Check sheet for the modelled part. Datum: model origin and axes. Units: mm. A direction names the side the tool comes from. Give positions to 0.01 mm unless a question says otherwise; leave off trailing zeros. Order: outer loops, then holes, each group sorted by start corner. A loop starts at its lowest first (then second) coordinate and runs counter-clockwise, first axis right, second up. Notation, with made-up numbers: (68.5, 40) -> (111.5, 40) arc R26 cw to (111.5, 64) -> close; hole circle Ø4 at (73.25, 88). An arc over 180 degrees is marked (long way). Answer in a Markdown table with one row per item. Add a question column.
(1) Thickness scan on L1, parallel to Y at x = 0, z = 1.5; L2, parallel to Z at x = -12.5, y = 11; L3, parallel to X at y = 5.25, z = 7. Record the ranges inside material, lowest first. Write a range as [from, to].
(2) Cross-section at B-B (y = 0). Record the cut outline in (x, z), then the cut area to 3 significant figures.
(3) Cross-section at C-C (z = 13). Record the cut outline in (x, y).
(4) Release check for a two-part mould opening along Z. For faces 1 (the face through (0, -12, 7)), 2 (the face through (-0.54, -2.44, 12.17)) record: released by +Z, released by -Z, zero draft, split by the parting line, or undercut.
(5) Set-up check for faces 3 (the face through (-1.84, -8.3, 19.07)), 4 (the face through (-2.437, 13.786, 7.07)), 5 (the face through (13.154, 4.794, 7.07)), 6 (the face through (-10.414, -5.964, 6.93)): record each of +Z, -Z, +X, -X, +Y, -Y from which the full face is reachable in a straight line by a thin tool's end or side.
(6) Cross-section at D-D (y = 6.5). Record the cut outline in (x, z).
(7) Cross-section at A-A (x = 0). Record the cut outline in (y, z).
(8) Go/stop test with flat-tipped pins: pin 1 (4 mm diameter, centred on x = 0, y = 0, fed in from -Z); pin 2 (10 mm diameter, centred on x = -13, y = 12, fed in from +Z); pin 3 (3.5 mm diameter, centred on x = 0, z = 19, fed in from -Y); pin 4 (4 mm diameter, centred on x = -13.5, z = 11, fed in from -Y). Record where each tip stops, or that it passes through.
```python
from build123d import *

# Parameters (mm, degrees)
SKETCH1_R                 = 17
BOSS_EXTRUDE1_DEPTH       = 14
CUT_EXTRUDE2_REACH        = 29.821
SKETCH3_R                 = 2.5
BOSS_EXTRUDE2_START       = 10
SKETCH5_R                 = 8.5
SKETCH5_R_2               = 2.5
BOSS_EXTRUDE2_DEPTH       = 10
SKETCH7_R                 = 17
SKETCH7_R_2               = 14
CUT_EXTRUDE5_DEPTH        = 5
SKETCH8_R                 = 2
CUT_EXTRUDE6_DEPTH        = 5
SKETCH9_R                 = 2
CUT_EXTRUDE7_DEPTH        = 10
M4_TAPPED_HOLE2_OUTLINE_W = 1.65
M4_TAPPED_HOLE2_OUTLINE_H = 10.992017373


with BuildPart() as part:
    # Sketch1 → Boss-Extrude1 (new body)
    with BuildSketch(Plane.XY):
        Circle(SKETCH1_R)
    extrude(amount=BOSS_EXTRUDE1_DEPTH)

    # Sketch3 → Cut-Extrude2 (cut, up to next)
    with BuildSketch(Plane.XY.offset(14), mode=Mode.PRIVATE) as cut_extrude2_sk1:
        Circle(SKETCH3_R)
    cut_extrude2_tool1 = extrude(cut_extrude2_sk1.sketch, amount=-CUT_EXTRUDE2_REACH, mode=Mode.PRIVATE) & part.part
    add(cut_extrude2_tool1.solids().sort_by_distance((0, 0, 14))[0], mode=Mode.SUBTRACT)

    # Sketch5 → Boss-Extrude2 (add)
    with BuildSketch(Plane.XY.offset(14).offset(BOSS_EXTRUDE2_START)):
        Circle(SKETCH5_R)
        Circle(SKETCH5_R_2, mode=Mode.SUBTRACT)
    extrude(amount=-BOSS_EXTRUDE2_DEPTH)

    # Sketch7 → Cut-Extrude5 (cut, symmetric)
    with BuildSketch(Plane(origin=(0, 0, 7), x_dir=(-1, 0, 0), z_dir=(0, 0, -1))):
        Circle(SKETCH7_R)
        Circle(SKETCH7_R_2, mode=Mode.SUBTRACT)
    extrude(amount=CUT_EXTRUDE5_DEPTH, both=True, mode=Mode.SUBTRACT)

    # Sketch8 → Cut-Extrude6 (cut, symmetric)
    with BuildSketch(Plane(origin=(0, 0, 7), x_dir=(-1, 0, 0), z_dir=(0, 0, -1))):
        with Locations((0, 14)):
            Circle(SKETCH8_R)
        with Locations((4.788282007, 13.155696691)):
            Circle(SKETCH8_R)
        with Locations((8.999026536, 10.724622204)):
            Circle(SKETCH8_R)
        with Locations((12.124355653, 7)):
            Circle(SKETCH8_R)
        with Locations((13.787308542, 2.431074487)):
            Circle(SKETCH8_R)
        with Locations((13.787308542, -2.431074487)):
            Circle(SKETCH8_R)
        with Locations((12.124355653, -7)):
            Circle(SKETCH8_R)
        with Locations((8.999026536, -10.724622204)):
            Circle(SKETCH8_R)
        with Locations((4.788282007, -13.155696691)):
            Circle(SKETCH8_R)
        with Locations((0, -14)):
            Circle(SKETCH8_R)
        with Locations((-4.788282007, -13.155696691)):
            Circle(SKETCH8_R)
        with Locations((-8.999026536, -10.724622204)):
            Circle(SKETCH8_R)
        with Locations((-12.124355653, -7)):
            Circle(SKETCH8_R)
        with Locations((-13.787308542, -2.431074487)):
            Circle(SKETCH8_R)
        with Locations((-13.787308542, 2.431074487)):
            Circle(SKETCH8_R)
        with Locations((-12.124355653, 7)):
            Circle(SKETCH8_R)
        with Locations((-8.999026536, 10.724622204)):
            Circle(SKETCH8_R)
        with Locations((-4.788282007, 13.155696691)):
            Circle(SKETCH8_R)
    extrude(amount=CUT_EXTRUDE6_DEPTH, both=True, mode=Mode.SUBTRACT)

    # Sketch9 → Cut-Extrude7 (cut)
    with BuildSketch(Plane(origin=(0, 0, 0), x_dir=(1, 0, 0), z_dir=(0, 1, 0))):
        with Locations(Location((0, -19, 0), (0, 0, 90))):
            Circle(SKETCH9_R)
    extrude(amount=CUT_EXTRUDE7_DEPTH, mode=Mode.SUBTRACT)

    # M4 Tapped Hole2: read off the stored shape, not the designer's step
    # M4 Tapped Hole2 outline → M4 Tapped Hole2 (revolve, cut)
    with BuildSketch(Plane.XY.offset(7)):
        with Locations((0.825, 7.373848872)):
            Rectangle(M4_TAPPED_HOLE2_OUTLINE_W, M4_TAPPED_HOLE2_OUTLINE_H)
    revolve(axis=Axis((0, 0, 7), (0, 1, 0)), mode=Mode.SUBTRACT)


solid = part.part
```
Answer below:
| question | item | result |
|---|---|---|
| 1 | L1 | y = [-17, -2.5], [2.5, 17] |
| 1 | L2 | z = [0, 2], [12, 14] |
| 1 | L3 | x = [-11.16, -1.65], [1.65, 11.16] |
| 2 | outline | (-17, 0) -> (-2.5, 0) -> (-2.5, 24) -> (-8.5, 24) -> (-8.5, 14) -> (-17, 14) -> (-17, 12) -> (-14, 12) -> (-14, 2) -> (-17, 2) -> close; (2.5, 0) -> (17, 0) -> (17, 2) -> (14, 2) -> (14, 12) -> (17, 12) -> (17, 14) -> (8.5, 14) -> (8.5, 24) -> (2.5, 24) -> close |
| 2 | area | 466 mm² |
| 3 | outline | circle Ø34 at (0, 0); hole circle Ø5 at (0, 0) |
| 4 | face 1 | undercut |
| 4 | face 2 | zero draft |
| 5 | face 3 | +Z |
| 5 | face 4 | -X, +Y |
| 5 | face 5 | +X, +Y |
| 5 | face 6 | none |
| 6 | outline | (-15.71, 0) -> (15.71, 0) -> (15.71, 2) -> (10.19, 2) -> (10.19, 12) -> (15.71, 12) -> (15.71, 14) -> (5.48, 14) -> (5.48, 24) -> (-5.48, 24) -> (-5.48, 14) -> (-15.71, 14) -> (-15.71, 12) -> (-10.19, 12) -> (-10.19, 2) -> (-15.71, 2) -> close; hole circle Ø4 at (0, 19); hole circle Ø3.3 at (0, 7) |
| 7 | outline | (-17, 0) -> (-2.5, 0) -> (-2.5, 24) -> (-8.5, 24) -> (-8.5, 14) -> (-17, 14) -> (-17, 12) -> (-12, 12) -> (-12, 2) -> (-17, 2) -> close; (2.5, 0) -> (17, 0) -> (17, 2) -> (12, 2) -> (12, 5.35) -> (2.5, 5.35) -> close; (2.5, 8.65) -> (12, 8.65) -> (12, 12) -> (17, 12) -> (17, 14) -> (8.5, 14) -> (8.5, 17) -> (2.5, 17) -> close; (2.5, 21) -> (8.5, 21) -> (8.5, 24) -> (2.5, 24) -> close |
| 8 | pin 1 | passes through |
| 8 | pin 2 | stops at z = 14 |
| 8 | pin 3 | stops at y = -8.5 |
| 8 | pin 4 | stops at y = -12.27 |
